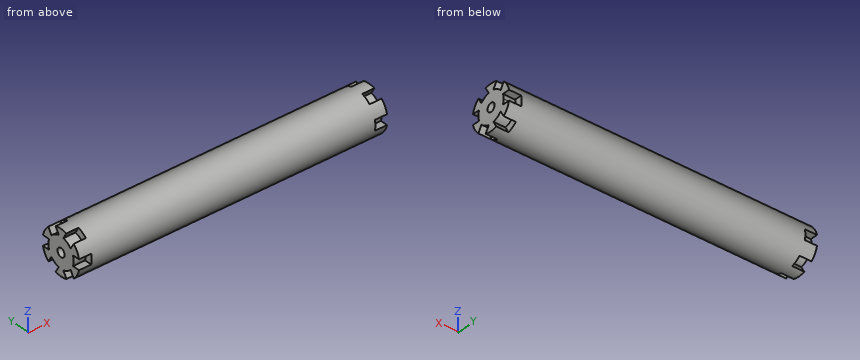
```python
from build123d import *

# Parameters (mm, degrees)
SKETCH1_R           = 22
SKETCH1_R_2         = 4.25
BOSS_EXTRUDE1_DEPTH = 305
CUT_EXTRUDE1_DEPTH  = 12
CUT_EXTRUDE2_START  = -293
CUT_EXTRUDE2_DEPTH  = 12


with BuildPart() as part:
    # Sketch1 → Boss-Extrude1 (new body)
    with BuildSketch(Plane(origin=(0, 0, 0), x_dir=(0, 0, -1), z_dir=(1, 0, 0))):
        Circle(SKETCH1_R)
        Circle(SKETCH1_R_2, mode=Mode.SUBTRACT)
    extrude(amount=BOSS_EXTRUDE1_DEPTH)

    # Sketch2 → Cut-Extrude1 (cut)
    with BuildSketch(Plane.ZY):
        with BuildLine():
            Line((16.053975315, 15.042269662), (9.747448714, 11.401194831))
            ThreePointArc((9.747448714, 11.401194831), (12.990381057, 7.5), (14.747448714, 2.740940793))
            Line((14.747448714, 2.740940793), (21.053975315, 6.382015624))
            ThreePointArc((21.053975315, 6.382015624), (19.052558883, 11), (16.053975315, 15.042269662))
        make_face()
        with BuildLine():
            Line((21.053975315, -6.382015624), (14.747448714, -2.740940793))
            ThreePointArc((14.747448714, -2.740940793), (12.990381057, -7.5), (9.747448714, -11.401194831))
            Line((9.747448714, -11.401194831), (16.053975315, -15.042269662))
            ThreePointArc((16.053975315, -15.042269662), (19.052558883, -11), (21.053975315, -6.382015624))
        make_face()
        with BuildLine():
            ThreePointArc((5, -14.142135624), (0, -15), (-5, -14.142135624))
            Line((-5, -14.142135624), (-5, -21.424285286))
            ThreePointArc((-5, -21.424285286), (0, -22), (5, -21.424285286))
            Line((5, -21.424285286), (5, -14.142135624))
        make_face()
        with BuildLine():
            ThreePointArc((-9.747448714, -11.401194831), (-12.990381057, -7.5), (-14.747448714, -2.740940793))
            Line((-14.747448714, -2.740940793), (-21.053975315, -6.382015624))
            ThreePointArc((-21.053975315, -6.382015624), (-19.052558883, -11), (-16.053975315, -15.042269662))
            Line((-16.053975315, -15.042269662), (-9.747448714, -11.401194831))
        make_face()
        with BuildLine():
            ThreePointArc((-14.747448714, 2.740940793), (-12.990381057, 7.5), (-9.747448714, 11.401194831))
            Line((-9.747448714, 11.401194831), (-16.053975315, 15.042269662))
            ThreePointArc((-16.053975315, 15.042269662), (-19.052558883, 11), (-21.053975315, 6.382015624))
            Line((-21.053975315, 6.382015624), (-14.747448714, 2.740940793))
        make_face()
        with BuildLine():
            Line((0, 22), (0, 15))
            ThreePointArc((0, 15), (2.536529681, 14.783978395), (5, 14.142135624))
            Line((5, 14.142135624), (5, 21.424285286))
            ThreePointArc((5, 21.424285286), (2.516517804, 21.85559741), (0, 22))
        make_face()
        with BuildLine():
            ThreePointArc((-5, 14.142135624), (-2.536529681, 14.783978395), (0, 15))
            Line((0, 15), (0, 22))
            ThreePointArc((0, 22), (-2.516517804, 21.85559741), (-5, 21.424285286))
            Line((-5, 21.424285286), (-5, 14.142135624))
        make_face()
    extrude(amount=-CUT_EXTRUDE1_DEPTH, mode=Mode.SUBTRACT)

    # Sketch2<4> → Cut-Extrude2 (cut)
    with BuildSketch(Plane.ZY.offset(CUT_EXTRUDE2_START)):
        with BuildLine():
            Line((16.053975315, 15.042269662), (9.747448714, 11.401194831))
            ThreePointArc((9.747448714, 11.401194831), (12.990381057, 7.5), (14.747448714, 2.740940793))
            Line((14.747448714, 2.740940793), (21.053975315, 6.382015624))
            ThreePointArc((21.053975315, 6.382015624), (19.052558883, 11), (16.053975315, 15.042269662))
        make_face()
        with BuildLine():
            Line((0, 22), (0, 15))
            ThreePointArc((0, 15), (2.536529681, 14.783978395), (5, 14.142135624))
            Line((5, 14.142135624), (5, 21.424285286))
            ThreePointArc((5, 21.424285286), (2.516517804, 21.85559741), (0, 22))
        make_face()
        with BuildLine():
            ThreePointArc((-5, 14.142135624), (-2.536529681, 14.783978395), (0, 15))
            Line((0, 15), (0, 22))
            ThreePointArc((0, 22), (-2.516517804, 21.85559741), (-5, 21.424285286))
            Line((-5, 21.424285286), (-5, 14.142135624))
        make_face()
        with BuildLine():
            ThreePointArc((-14.747448714, 2.740940793), (-12.990381057, 7.5), (-9.747448714, 11.401194831))
            Line((-9.747448714, 11.401194831), (-16.053975315, 15.042269662))
            ThreePointArc((-16.053975315, 15.042269662), (-19.052558883, 11), (-21.053975315, 6.382015624))
            Line((-21.053975315, 6.382015624), (-14.747448714, 2.740940793))
        make_face()
        with BuildLine():
            ThreePointArc((-9.747448714, -11.401194831), (-12.990381057, -7.5), (-14.747448714, -2.740940793))
            Line((-14.747448714, -2.740940793), (-21.053975315, -6.382015624))
            ThreePointArc((-21.053975315, -6.382015624), (-19.052558883, -11), (-16.053975315, -15.042269662))
            Line((-16.053975315, -15.042269662), (-9.747448714, -11.401194831))
        make_face()
        with BuildLine():
            ThreePointArc((5, -14.142135624), (0, -15), (-5, -14.142135624))
            Line((-5, -14.142135624), (-5, -21.424285286))
            ThreePointArc((-5, -21.424285286), (0, -22), (5, -21.424285286))
            Line((5, -21.424285286), (5, -14.142135624))
        make_face()
        with BuildLine():
            Line((21.053975315, -6.382015624), (14.747448714, -2.740940793))
            ThreePointArc((14.747448714, -2.740940793), (12.990381057, -7.5), (9.747448714, -11.401194831))
            Line((9.747448714, -11.401194831), (16.053975315, -15.042269662))
            ThreePointArc((16.053975315, -15.042269662), (19.052558883, -11), (21.053975315, -6.382015624))
        make_face()
    extrude(amount=-CUT_EXTRUDE2_DEPTH, mode=Mode.SUBTRACT)


solid = part.part
```
Model file for the job. Use its own axes, mm. Give positions to 0.01 mm unless a question says otherwise; leave off trailing zeros. Loops run counter-clockwise (first coordinate to the right, second up) from the corner with the lowest first, then second, coordinate; pieces in that order, holes last. Notation, with made-up numbers: (11.5, 37) -> (41.5, 37) arc R25 cw to (41.5, 50) -> close; hole circle Ø2 at (16.5, 51). An arc over 180 degrees is marked (long way). Use CSV: the item, a comma, the result in double quotes. Start each with the question number.
1) Flat gauge pins, fed straight in: pin 1 Ø2 at (x, y) = (208.5, -12.5) entering from -Z (3 decimals); pin 2 Ø6 at (x, z) = (65, -14) entering from +Y; pin 3 Ø12.5 at (y, z) = (6, -16.5) entering from +X; pin 4 Ø2.5 at (y, z) = (19.5, -1.5) entering from +X. Where does each tip first touch, or does it go through?
2) Slice it at B-B on x = 188. Give the cut face in (y, z), plus the area to 3 significant figures.
3) Slice it at A-A on y = 0. Give the cut face in (x, z), plus the area to 3 significant figures.
4) Wall check: line 1 (Z direction, x = 229, y = -0.5); line 2 (X direction, y = 19, z = 2); line 3 (Y direction, x = 35, z = 1). Give the ranges that are in metal, low to high.
Computed values:
1,pin 1,"stops at z = -18.755"
1,pin 2,"stops at y = 19.05"
1,pin 3,"stops at x = 305"
1,pin 4,"stops at x = 293"
2,outline,"circle Ø44 at (0, 0); hole circle Ø8.5 at (0, 0)"
2,area,"1,460 mm^2"
3,outline,"(0, -22) -> (305, -22) -> (305, -4.25) -> (0, -4.25) -> close; (0, 4.25) -> (305, 4.25) -> (305, 22) -> (0, 22) -> close"
3,area,"10,800 mm^2"
4,line 1,"z = -21.99 to -4.22, 4.22 to 21.99"
4,line 2,"x = 12 to 293"
4,line 3,"y = -21.98 to -4.13, 4.13 to 21.98"
